from build123d import *

# Parameters (mm, degrees)
SKETCH1_R           = 3.075
BOSS_EXTRUDE1_DEPTH = 5.842
FILLET1_R           = 6.35
SKETCH2_R           = 0.1984375
CUT_EXTRUDE1_DEPTH  = 53.014369063


with BuildPart() as part:
    # Sketch1 → Boss-Extrude1 (new body)
    with BuildSketch(Plane.XY):
        with BuildLine():
            Line((12.7, -12.7), (6.35, -12.7))
            Line((6.35, -12.7), (6.35, -18.542))
            Line((6.35, -18.542), (-6.35, -18.542))
            Line((-6.35, -18.542), (-6.35, -12.7))
            Line((-6.35, -12.7), (-12.7, -12.7))
            Line((-12.7, -12.7), (-12.7, -28.575))
            Line((-12.7, -28.575), (18.716430351, -37.605733858))
            ThreePointArc((18.716430351, -37.605733858), (30.161479232, -35.314751505), (34.902776944, -24.649019461))
            Line((34.902776944, -24.649019461), (31.75, 28.575))
            Line((31.75, 28.575), (-12.7, 28.575))
            Line((-12.7, 28.575), (-12.7, 12.7))
            Line((-12.7, 12.7), (-6.35, 12.7))
            Line((-6.35, 12.7), (-6.35, 18.542))
            Line((-6.35, 18.542), (6.35, 18.542))
            Line((6.35, 18.542), (6.35, 12.7))
            Line((6.35, 12.7), (12.7, 12.7))
            Line((12.7, 12.7), (12.7, 6.35))
            Line((12.7, 6.35), (18.542, 6.35))
            Line((18.542, 6.35), (18.542, -6.35))
            Line((18.542, -6.35), (12.7, -6.35))
            Line((12.7, -6.35), (12.7, -12.7))
        make_face()
        with Locations((22.225, -25.4)):
            Circle(SKETCH1_R, mode=Mode.SUBTRACT)
    extrude(amount=BOSS_EXTRUDE1_DEPTH)

    # Fillet1
    fillet1_edges = [part.edges().sort_by_distance(p)[0] for p in [
        (-12.7, 28.575, 2.921),
        (31.75, 28.575, 2.921),
        (-12.7, -28.575, 2.921),
    ]]
    fillet(fillet1_edges, radius=FILLET1_R)

    # Sketch2 → Cut-Extrude1 (cut, through all)
    with BuildSketch(Plane.XY.offset(5.842)):
        with Locations((12.7, 12.7)):
            Circle(SKETCH2_R)
        with Locations((12.7, -12.7)):
            Circle(SKETCH2_R)
    extrude(amount=-CUT_EXTRUDE1_DEPTH, mode=Mode.SUBTRACT)


solid = part.part
Here's how the part is built. I have some questions about the finished solid (model axes, mm). A direction names the side the tool comes from. Coordinates: 2 decimals unless noted, no trailing zeros. Order: outer loops, then holes, each group sorted by start corner. A loop starts at its lowest first (then second) coordinate and runs counter-clockwise, first axis right, second up. Notation, with made-up numbers: M 75,60 L 94,60 A18 cw 94,74 Z; hole C 80,36.25 d8. An arc over 180 degrees is marked long. Answer as CSV lines item,"result". Start each with the question number.
1. I need wall thicknesses on line 1 (Y direction, x = 9.5, z = 2.9) (3 decimals); line 2 (X direction, y = -13, z = 3.05); line 3 (X direction, y = 18.5, z = 2.1). Which ranges of each line are inside material? Lowest first, please. Write a range as [from, to].
2. We'd pull the mould along X, two halves only. Please class faces 4 (the flat face through (12.7, 9, 3)), 5 (the flat face through (21, -4, 0)), 6 (the flat face through (6.35, -16, 3)): released by +X, released by -X, zero draft, split by the parting line, or undercut.
3. On a 3-axis mill with a long thin cutter (end or side, diameter ignored), from which of +Z, -Z, +X, -X, +Y, -Y can I reach the whole of each face in a straight line? I mean faces 1 (the flat face through (-10, 12.7, 3)), 2 (the flat face through (-12.7, 18, 3)), 3 (the flat face through (-6.35, -16, 3)). Say none if no direction works.
4. For pin 1 (3 mm diameter, centred on y = 14.5, z = 2.5, fed in from +X); pin 2 (1.8 mm diameter, centred on x = 0, z = 2.5, fed in from -Y); pin 3 (1.8 mm diameter, centred on x = 15, z = 1.5, fed in from -Y), each with a flat end and sliding along its axis, tell me the tip position at first contact or that it passes through.
5. I want a section at D-D, the plane y = 8.5. Write out the boundary of the cut face in (x, z).
6. I want a section at C-C, the plane y = -25.4. Write out the boundary of the cut face in (x, z) (3 decimals), and give its area (3 significant figures).
7. I want a section at B-B, the plane x = 16.5. Write out the boundary of the cut face in (y, z) (3 decimals), and give its area (3 significant figures).
Recorded:
1,line 1,"y = [-34.956, -12.7], [12.7, 28.575]"
1,line 2,"x = [-12.7, -6.35], [6.35, 34.21]"
1,line 3,"x = [-12.7, -6.35], [6.35, 32.35]"
2,face 4,"released by -X"
2,face 5,"zero draft"
2,face 6,"undercut"
3,face 1,"+Z, -Z, -X"
3,face 2,"+Z, -Z, -X, +Y, -Y"
3,face 3,"+Z, -Z"
4,pin 1,"stops at x = 32.67"
4,pin 2,"stops at y = -32.48"
4,pin 3,"stops at y = -36.8"
5,outline,"M 12.7,0 L 32.94,0 L 32.94,5.84 L 12.7,5.84 Z"
6,outline,"M -12.493,0 L 19.15,0 L 19.15,5.842 L -12.493,5.842 Z; M 25.3,0 L 34.925,0 L 34.925,5.842 L 25.3,5.842 Z"
6,area,"241 mm2"
7,outline,"M -36.969,0 L -6.35,0 L -6.35,5.842 L -36.969,5.842 Z; M 6.35,0 L 28.575,0 L 28.575,5.842 L 6.35,5.842 Z"
7,area,"309 mm2"
